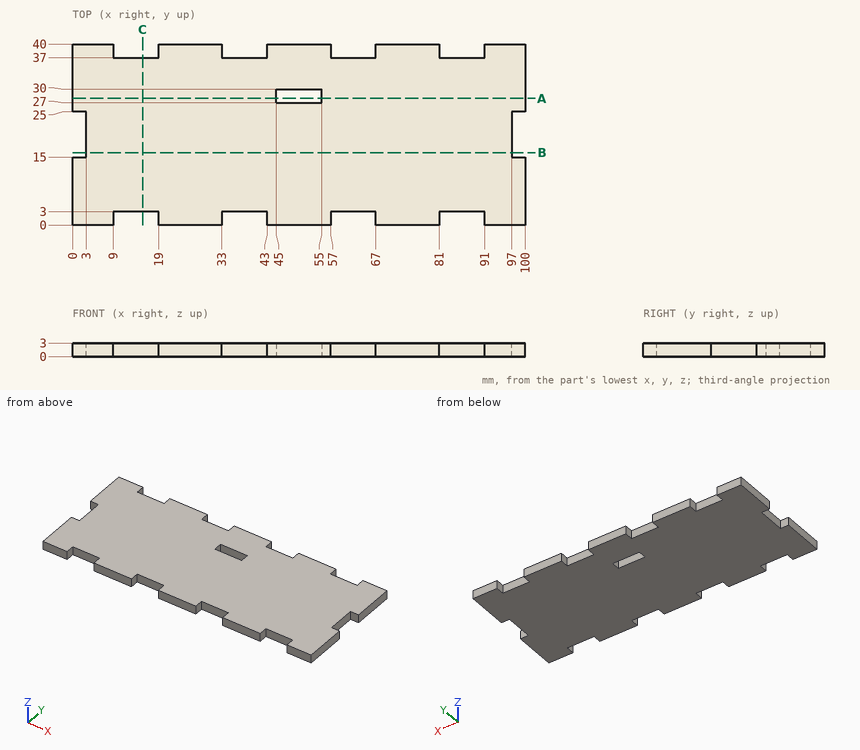
Input: dimensioned drawing with shaded views. Units: mm. Origin: part minimum x, y, z. Coordinates: 2 decimals unless noted, no trailing zeros. Loops run counter-clockwise (first coordinate to the right, second up) from the corner with the lowest first, then second, coordinate; pieces in that order, holes last. Notation, with made-up numbers: M -23,63.5 L 16,63.5 A16 cw 16,87.5 Z; hole C 88,5.5 d6. An arc over 180 degrees is marked long. Use a Markdown table: item, result. Add a question column.
Q1. Section query B-B, the plane y = 16. Return loops of the section in (x, z), and give its area (3 significant figures).
Q2. Material intervals for L1, parallel to X at y = 24.5, z = 1.95; L2, parallel to Y at x = 38, z = 0.2; L3, parallel to Y at x = 51.5, z = 1.25, sorted ascending.
Q3. First-contact query: pin 1 (0.9 mm diameter, centred on y = 18.5, z = 1.5, fed in from +X); pin 2 (0.9 mm diameter, centred on x = 39, z = 2, fed in from -Y). Flat tips, straight axial feed; report the tip coordinate or a pass-through.
Q4. Section query C-C, the plane x = 15.5. Return loops of the section in (y, z), and give its area (3 significant figures).
Q5. Section query A-A, the plane y = 28. Return loops of the section in (x, z).
Result:
| question | item | result |
|---|---|---|
| 1 | outline | M 3,0 L 97,0 L 97,3 L 3,3 Z |
| 1 | area | 282 mm2 |
| 2 | L1 | x = 3 to 97 |
| 2 | L2 | y = 3 to 37 |
| 2 | L3 | y = 0 to 27, 30 to 40 |
| 3 | pin 1 | stops at x = 97 |
| 3 | pin 2 | stops at y = 3 |
| 4 | outline | M 3,0 L 37,0 L 37,3 L 3,3 Z |
| 4 | area | 102 mm2 |
| 5 | outline | M 0,0 L 45,0 L 45,3 L 0,3 Z; M 55,0 L 100,0 L 100,3 L 55,3 Z |
